```python
from build123d import *

# Parameters (mm, degrees)
ESQUISSE1_W             = 40
ESQUISSE1_H             = 45
ESQUISSE1_R             = 1.75
BOSS_EXTRU_1_DEPTH      = 10
ESQUISSE2_R             = 4
ENL_V_MAT_EXTRU_2_DEPTH = 5
BOSS_EXTRU_2_DEPTH      = 10
ESQUISSE4_W             = 5
ESQUISSE4_H             = 50
BOSS_EXTRU_3_DEPTH      = 20
ENL_V_MAT_EXTRU_3_REACH = 106.163
ESQUISSE5_R             = 3.25
ESQUISSE8_R             = 2.75
BOSS_EXTRU_8_DEPTH      = 10
ENL_V_MAT_EXTRU_5_REACH = 114.472
ESQUISSE9_R             = 15
CHANFREIN2_SIZE         = 15
ENL_V_MAT_EXTRU_4_REACH = 104.103
CHANFREIN3_SIZE         = 3.5
BOSS_EXTRU_4_DEPTH      = 5


# Some blends are built 0.0001 mm under size
with BuildPart() as part:
    # Esquisse1 → Boss.-Extru.1 (new body)
    with BuildSketch(Plane.XY):
        with Locations((-20, 22.5)):
            Rectangle(ESQUISSE1_W, ESQUISSE1_H)
        with Locations((-3.5, 32.5)):
            Circle(ESQUISSE1_R, mode=Mode.SUBTRACT)
        with Locations((-23.5, 32.5)):
            Circle(ESQUISSE1_R, mode=Mode.SUBTRACT)
        with Locations((-23.5, 12.5)):
            Circle(ESQUISSE1_R, mode=Mode.SUBTRACT)
        with Locations((-3.5, 12.5)):
            Circle(ESQUISSE1_R, mode=Mode.SUBTRACT)
    extrude(amount=BOSS_EXTRU_1_DEPTH)

    # Esquisse2 → Enlèv. mat.-Extru.2 (cut)
    with BuildSketch(Plane.XY.offset(10)):
        with Locations((-23.5, 32.5)):
            Circle(ESQUISSE2_R)
        with Locations((-3.5, 32.5)):
            Circle(ESQUISSE2_R)
        with Locations((-23.5, 12.5)):
            Circle(ESQUISSE2_R)
        with Locations((-3.5, 12.5)):
            Circle(ESQUISSE2_R)
    extrude(amount=-ENL_V_MAT_EXTRU_2_DEPTH, mode=Mode.SUBTRACT)

    # Esquisse3 → Boss.-Extru.2 (add)
    with BuildSketch(Plane.ZY.offset(40)):
        Polygon((10, 0), (45, 35), (45, 85), (40, 85), (0, 45), (10, 45), align=None)
    extrude(amount=-BOSS_EXTRU_2_DEPTH)

    # Esquisse4 → Boss.-Extru.3 (add)
    with BuildSketch(Plane(origin=(-30, 0, 0), x_dir=(0, 0, -1), z_dir=(1, 0, 0))):
        with Locations((-42.5, 60)):
            Rectangle(ESQUISSE4_W, ESQUISSE4_H)
    extrude(amount=BOSS_EXTRU_3_DEPTH)

    # Esquisse5 → Enlèv. mat.-Extru.3 (cut, up to next)
    with BuildSketch(Plane.XY.offset(45), mode=Mode.PRIVATE) as enl_v_mat_extru_3_sk1:
        with Locations((-18.5, 70)):
            Circle(ESQUISSE5_R)
    enl_v_mat_extru_3_tool1 = extrude(enl_v_mat_extru_3_sk1.sketch, amount=-ENL_V_MAT_EXTRU_3_REACH, mode=Mode.PRIVATE) & part.part
    # Esquisse5 → Enlèv. mat.-Extru.3 (cut, up to next)
    with BuildSketch(Plane.XY.offset(45), mode=Mode.PRIVATE) as enl_v_mat_extru_3_sk2:
        with Locations((-18.5, 50)):
            Circle(ESQUISSE5_R)
    enl_v_mat_extru_3_tool2 = extrude(enl_v_mat_extru_3_sk2.sketch, amount=-ENL_V_MAT_EXTRU_3_REACH, mode=Mode.PRIVATE) & part.part
    add(enl_v_mat_extru_3_tool1.solids().sort_by_distance((-18.5, 70, 45))[0], mode=Mode.SUBTRACT)
    add(enl_v_mat_extru_3_tool2.solids().sort_by_distance((-18.5, 50, 45))[0], mode=Mode.SUBTRACT)

    # Esquisse8 → Boss.-Extru.8 (add)
    with BuildSketch(Plane.XZ):
        Polygon((3.3834406, 0), (-40, 0), (-40, 10), (-30, 10), (-8.6165594, 29), (3.3834406, 29), align=None)
        with Locations(Location((-2.6165594, 22, 0), (0, 0, 270))):
            Circle(ESQUISSE8_R, mode=Mode.SUBTRACT)
    extrude(amount=BOSS_EXTRU_8_DEPTH)

    # Esquisse9 → Enlèv. mat.-Extru.5 (cut, up to next)
    with BuildSketch(Plane.XZ.offset(10), mode=Mode.PRIVATE) as enl_v_mat_extru_5_sk1:
        with Locations((16.3834406, 22)):
            Circle(ESQUISSE9_R)
    enl_v_mat_extru_5_tool1 = extrude(enl_v_mat_extru_5_sk1.sketch, amount=-ENL_V_MAT_EXTRU_5_REACH, mode=Mode.PRIVATE) & part.part
    add(enl_v_mat_extru_5_tool1.solids().sort_by_distance((16.383441, -10, 22))[0], mode=Mode.SUBTRACT)

    # Chanfrein2
    # the kernel refuses this chamfer: 15 mm, written as the material it adds along each edge
    with BuildSketch(Plane(origin=(-30, 83.575244819, 10), x_dir=(1, 0, 0), z_dir=(0, -1, 0))) as chanfrein2_piece_1_section:
        Polygon((CHANFREIN2_SIZE, 0), (0, CHANFREIN2_SIZE), (0, 0), align=None)
    chanfrein2_piece_1 = extrude(amount=122.150489639, mode=Mode.PRIVATE)
    chanfrein2_piece_1 = split(chanfrein2_piece_1, bisect_by=Plane(origin=(-30, 69.28762241, 24.28762241), z_dir=(0, -0.707106781186543, 0.7071067811865521)), keep=Keep.TOP, mode=Mode.PRIVATE)
    chanfrein2_piece_1 = chanfrein2_piece_1 - Plane(origin=(-23.5, 12.5, 10), x_dir=(1, 0, 0), z_dir=(0, 0, 1)) * Cylinder(4, 305, mode=Mode.PRIVATE)
    chanfrein2_piece_1 = chanfrein2_piece_1 - Plane(origin=(-23.5, 32.5, 10), x_dir=(1, 0, 0), z_dir=(0, 0, 1)) * Cylinder(4, 305, mode=Mode.PRIVATE)
    chanfrein2_piece_1 = split(chanfrein2_piece_1, bisect_by=Plane(origin=(-30, 41.78762241, 51.78762241), z_dir=(0, 0.7071067811865328, -0.7071067811865622)), keep=Keep.TOP, mode=Mode.PRIVATE)
    chanfrein2_piece_1 = split(chanfrein2_piece_1, bisect_by=Plane(origin=(-41.78762241, 71.78762241, 10), z_dir=(-0.7071067811865475, -0.7071067811865477, 0)), keep=Keep.TOP, mode=Mode.PRIVATE)
    add(chanfrein2_piece_1)
    with BuildSketch(Plane(origin=(-30, 83.575244819, 10), x_dir=(1, 0, 0), z_dir=(0, -1, 0))) as chanfrein2_piece_2_section:
        Polygon((CHANFREIN2_SIZE, 0), (0, CHANFREIN2_SIZE), (0, 0), align=None)
    chanfrein2_piece_2 = extrude(amount=122.150489639, mode=Mode.PRIVATE)
    chanfrein2_piece_2 = split(chanfrein2_piece_2, bisect_by=Plane(origin=(-30, -10, 10), z_dir=(0, 1, 0)), keep=Keep.TOP, mode=Mode.PRIVATE)
    chanfrein2_piece_2 = split(chanfrein2_piece_2, bisect_by=Plane(origin=(-30, 41.78762241, 51.78762241), z_dir=(0, -0.7071067811865328, 0.7071067811865622)), keep=Keep.TOP, mode=Mode.PRIVATE)
    chanfrein2_piece_2 = split(chanfrein2_piece_2, bisect_by=Plane(origin=(-30, 83.575244819, 10), z_dir=(0.66421730691086, 0, -0.7475395435694919)), keep=Keep.TOP, mode=Mode.PRIVATE)
    add(chanfrein2_piece_2)
    with BuildSketch(Plane(origin=(-30, 45, -38.575244819), x_dir=(1, 0, 0), z_dir=(0, 0, 1))) as chanfrein2_piece_3_section:
        Polygon((CHANFREIN2_SIZE, 0), (0, CHANFREIN2_SIZE), (0, 0), align=None)
    chanfrein2_piece_3 = extrude(amount=87.150489639, mode=Mode.PRIVATE)
    chanfrein2_piece_3 = split(chanfrein2_piece_3, bisect_by=Plane(origin=(-30, 25.71237759, -19.28762241), z_dir=(0, -0.707106781186543, 0.7071067811865521)), keep=Keep.TOP, mode=Mode.PRIVATE)
    chanfrein2_piece_3 = split(chanfrein2_piece_3, bisect_by=Plane(origin=(1.78762241, 45, -6.78762241), z_dir=(-0.7071067811865476, 0, -0.7071067811865476)), keep=Keep.TOP, mode=Mode.PRIVATE)
    add(chanfrein2_piece_3)
    with BuildSketch(Plane(origin=(-30, 35, 40), x_dir=(0, 0, -1), z_dir=(0, 1, 0))) as chanfrein2_piece_4_section:
        Polygon((CHANFREIN2_SIZE, 0), (0, -CHANFREIN2_SIZE), (0, 0), align=None)
    chanfrein2_piece_4 = extrude(amount=88.575244819, mode=Mode.PRIVATE)
    chanfrein2_piece_4 = split(chanfrein2_piece_4, bisect_by=Plane(origin=(-30, 60, 15), z_dir=(0, -0.707106781186543, 0.7071067811865521)), keep=Keep.TOP, mode=Mode.PRIVATE)
    chanfrein2_piece_4 = chanfrein2_piece_4 - Plane(origin=(-18.5, 70, 40), x_dir=(1, 0, 0), z_dir=(0, 0, 1)) * Cylinder(3.25, 238, mode=Mode.PRIVATE)
    chanfrein2_piece_4 = chanfrein2_piece_4 - Plane(origin=(-18.5, 50, 40), x_dir=(1, 0, 0), z_dir=(0, 0, 1)) * Cylinder(3.25, 238, mode=Mode.PRIVATE)
    add(chanfrein2_piece_4)

    # Esquisse6 → Enlèv. mat.-Extru.4 (cut, up to next)
    with BuildSketch(Plane(origin=(0, 0, 40), x_dir=(-1, 0, 0), z_dir=(0, 0, -1)), mode=Mode.PRIVATE) as enl_v_mat_extru_4_sk1:
        with BuildLine():
            Line((10.5, 70), (10.5, 85))
            Line((10.5, 85), (26.5, 85))
            Line((26.5, 85), (26.5, 70))
            ThreePointArc((26.5, 70), (18.5, 62), (10.5, 70))
        make_face()
    enl_v_mat_extru_4_tool1 = extrude(enl_v_mat_extru_4_sk1.sketch, amount=ENL_V_MAT_EXTRU_4_REACH, mode=Mode.PRIVATE) & part.part
    # Esquisse6 → Enlèv. mat.-Extru.4 (cut, up to next)
    with BuildSketch(Plane(origin=(0, 0, 40), x_dir=(-1, 0, 0), z_dir=(0, 0, -1)), mode=Mode.PRIVATE) as enl_v_mat_extru_4_sk2:
        with BuildLine():
            Line((10.5, 50), (10.5, 35))
            Line((10.5, 35), (26.5, 35))
            Line((26.5, 35), (26.5, 50))
            ThreePointArc((26.5, 50), (18.5, 58), (10.5, 50))
        make_face()
    enl_v_mat_extru_4_tool2 = extrude(enl_v_mat_extru_4_sk2.sketch, amount=ENL_V_MAT_EXTRU_4_REACH, mode=Mode.PRIVATE) & part.part
    add(enl_v_mat_extru_4_tool1.solids().sort_by_distance((-18.5, 74.283507, 40))[0], mode=Mode.SUBTRACT)
    add(enl_v_mat_extru_4_tool2.solids().sort_by_distance((-18.5, 45.716493, 40))[0], mode=Mode.SUBTRACT)

    # Chanfrein3
    chanfrein3_edges = [part.edges().sort_by_distance(p)[0] for p in [
        (-30, 35, 35),
    ]]
    chamfer(chanfrein3_edges, length=CHANFREIN3_SIZE - 0.0001)  # a hair under: the kernel refuses the full size

    # Esquisse7 → Boss.-Extru.4 (add)
    with BuildSketch(Plane.ZY.offset(40)):
        with BuildLine():
            Line((28.914213562, 18.914213562), (31.035533906, 21.035533906))
            ThreePointArc((31.035533906, 21.035533906), (31.035533906, 13.964466094), (23.964466094, 13.964466094))
            Line((23.964466094, 13.964466094), (26.085786438, 16.085786438))
            ThreePointArc((26.085786438, 16.085786438), (28.914213562, 16.085786438), (28.914213562, 18.914213562))
        make_face()
    extrude(amount=-BOSS_EXTRU_4_DEPTH)


solid = part.part
```
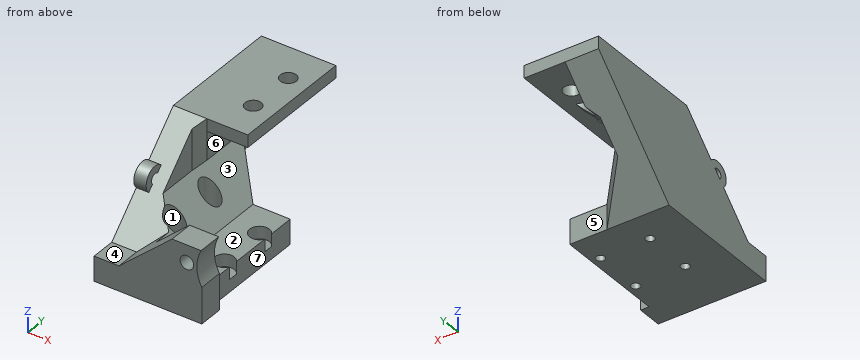
Verification items for the finished model (mm, model axes). Face numbers are marked on the shaded views. A direction names the side the tool comes from. Coordinates: 2 decimals unless noted, no trailing zeros. Write each loop counter-clockwise with the first axis right and the second up, starting at its lowest first coordinate (ties: lowest second). Pieces come first, ordered by that corner, then holes. Notation, with made-up numbers: M 47,1 L 51,1 A32 cw 51,37 Z; hole C 29,-12.75 d1. An arc over 180 degrees is marked long. One line per item, written item: value.
Item 1: Section check D-D, the plane y = 32.5. Record the boundary of the cut face in (x, z), plus the area to 3 significant figures.
Check sheet entries:
outline: M -40,0 L -25.25,0 L -25.25,5 L -27.5,5 L -27.5,22.5 L -30,25 L -29,26 L -29,42.5 L -40,42.5 Z; M -21.75,0 L -5.25,0 L -5.25,5 L -7.5,5 L -7.5,10 L -15,10 L -19.5,14.5 L -19.5,5 L -21.75,5 Z; M -1.75,0 L 0,0 L 0,5 L -1.75,5 Z
area: 674 mm^2
Item 2: Section check A-A, the plane y = 17.5. Record the boundary of the cut face in (x, z), plus the area to 4 significant figures.
Check sheet entries:
outline: M -40,0 L 0,0 L 0,10 L -15,10 L -30,25 L -30,27.5 L -40,27.5 Z; M -40,29.5 L -35,29.5 L -35,32.5 L -40,32.5 Z
area: 702.5 mm^2
Item 3: Section check B-B, the plane x = -18.5. Record the boundary of the cut face in (y, z).
Check sheet entries:
outline: M -10,0 L 45,0 L 48.5,3.5 L 48.5,13.5 L 0,13.5 L 0,20.22 L -10,20.22 Z; M 35,40 L 46.75,40 L 46.75,45 L 35,45 Z; M 53.25,40 L 58,40 L 58,36.5 L 62,36.5 L 62,40 L 66.75,40 L 66.75,45 L 53.25,45 Z; M 73.25,40 L 85,40 L 85,45 L 73.25,45 Z
Item 4: Section check C-C, the plane z = 27.5. Record the boundary of the cut face in (x, y), plus the area to 3 significant figures.
Check sheet entries:
outline: M -40,12.5 L -35,12.5 L -35,15.5 L -40,15.5 Z; M -40,17.5 L -30,17.5 L -30,31.5 L -27.5,34 L -27.5,72.5 L -40,72.5 Z; M -10.3,-10 L 2.43,-10 L 2.43,0 L -10.3,0 Z
area: 792 mm^2
Item 5: Gauge pin test, flat ends, axial feed: pin 1 Ø5 at (x, y) = (-3.5, 32.5) entering from +Z; pin 2 Ø4.5 at (x, y) = (-7, 13.5) entering from +Z; pin 3 Ø5 at (x, y) = (-21, 55.5) entering from -Z; pin 4 Ø3 at (y, z) = (70, 23) entering from -X. Record the tip position at first contact, or that the pin passes through.
Check sheet entries:
pin 1: stops at z = 5
pin 2: stops at z = 10
pin 3: stops at z = 31.65
pin 4: stops at x = -40
Item 6: Scan lines: line 1 along X through (y, z) = (12.5, 1.85); line 2 along Y through (x, z) = (-3.5, 8.65); line 3 along Y through (x, z) = (-23.5, 3.05). Record each from-to range of solid material in increasing order.
Check sheet entries:
line 1: x = -40 to -25.25, -21.75 to -5.25, -1.75 to 0
line 2: y = -10 to 8.5, 16.5 to 28.5, 36.5 to 45
line 3: y = -10 to 10.75, 14.25 to 30.75, 34.25 to 48.05
Item 7: Mould release check, pull along X, two halves, no side actions. Record for the marked faces 1, 2 and 3: pulls with the +X half, pulls with the -X half, needs draft (parallel to the pull), parting line crosses it, or undercut.
Check sheet entries:
face 1: undercut
face 2: needs draft
face 3: pulls with the +X half
Item 8: Access from +Z, -Z, +X, -X, +Y, -Y to the whole of each face (thin tool, end or side, straight path). Record for the marked faces 4, 5, 6 and 7.
Check sheet entries:
face 4: +Z, -X, -Y
face 5: -Z, +X, +Y
face 6: +X, -Y
face 7: +Z, -Z, +X, +Y
